Geometry: final body of the model. Coordinates: model frame, mm. A direction names the side the tool comes from. Coordinates: 2 decimals unless noted, no trailing zeros. Order: outer loops, then holes, each group sorted by start corner. A loop starts at its lowest first (then second) coordinate and runs counter-clockwise, first axis right, second up. Notation, with made-up numbers: (-35, 12) -> (15, 12) arc R23 ccw to (15, 48) -> close; hole circle Ø1 at (-22.5, -28.75). An arc over 180 degrees is marked (long way). Answer in a Markdown table with one row per item. Add a question column.
1) Section query B-B on y = -4.5. Return the cut outline in (x, z).
2) Ray query, line 1 (Z direction, x = -51.5, y = -8.5); line 2 (X direction, y = 7, z = -59.5); line 3 (X direction, y = -2.75, z = 29). Return the intervals inside material, ascending. Write a range as from..to.
3) Section query D-D on x = -47. Count the separate pieces of the cut face and the enclosed holes in it, then the cut area to 3 significant figures.
4) Pull-direction query (Z, two-part tool) for faces 1 (the face through (21.737, 1.568, -19.309)), 2 (the face through (-32.644, 0, 7)), 3 (the face through (-10.73, -11.17, 23.97)), 4 (the face through (-55.687, 0, -49)); classes: +Z half, -Z half, draft (parallel to the pull), parting line (faces both ways), or undercut.
5) Set-up query: faces 5 (the face through (-42.561, -11.172, -12.327)), 6 (the face through (-43.3, 2.4, -11.01)), 7 (the face through (5.96, 2.4, -1.27)). Return all of +Z, -Z, +X, -X, +Y, -Y with unobstructed straight access to the full face (end or side cutting, diameter ignored); none if empty.
6) Contact query for flat-ended pins moving along their axis: P1, Ø2, axis at x = -52, y = -6.5, coming from the -Z side; P2, Ø14.5, axis at y = 5.5, z = 26, coming from the +X side; P3, Ø2, axis at x = 0.5, z = 0.5, coming from the -Y side. Output: stop coordinate, or through.
7) Section query C-C on z = -69. Return the cut outline in (x, y).
8) Section query A-A on z = 18.5. Return the cut outline in (x, y), then the cut area to 3 significant figures.
```python
from build123d import *

# Parameters (mm, degrees)
F1_DEPTH = 12.7
F2_R     = 5.08


with BuildPart() as f1:
    # F0 (on Front) → F1 (new body, symmetric)
    with BuildSketch(Plane.XZ):
        Polygon((-42.56532, 53.124823), (-54.08676, 52.804779), (-54.08676, 43.843661), (-42.56532, 43.843661), align=None)
        Polygon((-38.601383, 32.591193), (-42.56532, 43.843661), (-62.407799, 14.399981), (-50.886359, 14.399981), align=None)
        Polygon((-9.281159, 15.680142), (-32.644082, 15.680142), (-32.644082, 0), (-55.686962, -23.803976), (-55.686962, -77.451505), (22.082759, -77.451505), (22.082759, -19.20422), align=None)
        Polygon((0, 53.124823), (-42.56532, 53.124823), (-42.56532, 43.843661), (-38.601383, 32.591193), (-32.644082, 15.680142), (-9.281159, 15.680142), (-9.281159, 33.922419), (12.112285, 33.922419), align=None)
    extrude(amount=F1_DEPTH, both=True)

    # F2
    f2_edges = [f1.edges().sort_by_distance(p)[0] for p in [
        (-55.686962, -12.7, -50.62774),
        (-44.165522, -12.7, -11.901988),
        (-55.686962, 0, -23.803976),
        (-55.686962, 12.7, -50.62774),
        (-55.686962, 0, -77.451505),
        (-16.802101, -12.7, -77.451505),
        (22.082759, -12.7, -48.327862),
        (6.4008, -12.7, -1.762039),
        (-9.281159, -12.7, 24.80128),
        (6.056143, -12.7, 43.523621),
        (-54.08676, -12.7, 48.32422),
        (-54.08676, 12.7, 48.32422),
        (-62.407799, 0, 14.399981),
        (22.082759, 12.7, -48.327862),
        (22.082759, 0, -19.20422),
        (22.082759, 0, -77.451505),
    ]]
    fillet(f2_edges, radius=F2_R)


solid = f1.part
```
Result:
| question | item | result |
|---|---|---|
| 1 | outline | (-57.07, 22.32) arc R5.08 ccw to (-52.86, 14.4) -> (-50.89, 14.4) -> (-38.6, 32.59) -> (-32.64, 15.68) -> (-32.64, 0) -> (-54.26, -22.33) arc R5.08 ccw to (-55.69, -25.86) -> (-55.69, -72.37) arc R5.08 ccw to (-50.61, -77.45) -> (17, -77.45) arc R5.08 ccw to (22.08, -72.37) -> (22.08, -21.15) arc R5.08 ccw to (20.78, -17.76) -> (-9.28, 15.68) -> (-9.28, 33.92) -> (12.11, 33.92) -> (0, 53.12) -> (-42.57, 53.12) -> (-54.09, 52.8) -> (-54.09, 43.84) -> (-42.57, 43.84) -> close |
| 2 | line 1 | -77.29..-19.59, 14.4..30.59, 43.84..52.88 |
| 2 | line 2 | -55.69..22.08 |
| 2 | line 3 | -52.57..-41.03, -37.34..-9.28 |
| 3 | separate pieces | 3 |
| 3 | enclosed holes | 0 |
| 3 | area | 2,240 mm2 |
| 4 | face 1 | +Z half |
| 4 | face 2 | undercut |
| 4 | face 3 | undercut |
| 4 | face 4 | draft |
| 5 | face 5 | -X, -Y |
| 5 | face 6 | -X, +Y, -Y |
| 5 | face 7 | +X, +Y, -Y |
| 6 | P1 | z = -77.44 |
| 6 | P2 | x = -9.28 |
| 6 | P3 | y = -12.56 |
| 7 | outline | (-55.69, -7.62) arc R5.08 ccw to (-50.61, -12.7) -> (17, -12.7) arc R5.08 ccw to (22.08, -7.62) -> (22.08, 7.62) arc R5.08 ccw to (17, 12.7) -> (-50.61, 12.7) arc R5.08 ccw to (-55.69, 7.62) -> close |
| 8 | outline | (-57.84, -12.7) -> (-48.12, -12.7) -> (-48.12, 12.7) -> (-57.84, 12.7) -> close; (-33.64, -12.7) -> (-14.36, -12.7) arc R5.08 ccw to (-9.28, -7.62) -> (-9.28, 12.7) -> (-33.64, 12.7) -> close |
| 8 | area | 860 mm2 |
